Source: CAD feature listing. Evaluate the final solid. Frame: model axes, mm. Give positions to 0.01 mm unless a question says otherwise; leave off trailing zeros. Loops run counter-clockwise (first coordinate to the right, second up) from the corner with the lowest first, then second, coordinate; pieces in that order, holes last. Notation, with made-up numbers: M 44.5,13.5 L 55.5,13.5 A16 ccw 55.5,32.5 Z; hole C 7,71.5 d1. An arc over 180 degrees is marked long. Answer in a Markdown table with one row per item.
```python
from build123d import *

# Parameters (mm, degrees)
EXTRUDE_THIN2_DEPTH = 222.25
FILLET1_R           = 1.27


with BuildPart() as part:
    # Sketch1 → Extrude-Thin2 (new body)
    with BuildSketch(Plane.XY):
        with BuildLine():
            Line((0, 22.225), (-5.55625, 22.225))
            ThreePointArc((-5.55625, 22.225), (-8.727268782, 18.891050689), (-5.23875, 15.890914887))
            Line((-5.23875, 15.890914887), (-5.23875, 12.715914887))
            Line((-5.23875, 12.715914887), (-1.27, 12.715914887))
            Line((-1.27, 12.715914887), (-1.27, 5.55625))
            ThreePointArc((-1.27, 5.55625), (-4.048125, 2.778125), (-1.27, 0))
            Line((-1.27, 0), (0, 0))
            Line((0, 0), (0, 1.27))
            Line((0, 1.27), (-1.27, 1.27))
            ThreePointArc((-1.27, 1.27), (-2.593079188, 3.501936079), (0, 3.591476717))
            Line((0, 3.591476717), (0, 13.985914887))
            Line((0, 13.985914887), (-3.96875, 13.985914887))
            Line((-3.96875, 13.985914887), (-3.96875, 17.996971629))
            ThreePointArc((-3.96875, 17.996971629), (-7.234797593, 18.1491654), (-5.55625, 20.955))
            Line((-5.55625, 20.955), (0, 20.955))
            Line((0, 20.955), (0, 22.225))
        make_face()
    extrude(amount=-EXTRUDE_THIN2_DEPTH)

    # Fillet1
    fillet1_edges = [part.edges().sort_by_distance(p)[0] for p in [
        (-5.23875, 12.715914887, -111.125),
        (-3.96875, 17.996971629, -111.125),
        (0, 13.985914887, -111.125),
        (0, 3.591476717, -111.125),
    ]]
    fillet(fillet1_edges, radius=FILLET1_R)


solid = part.part
```
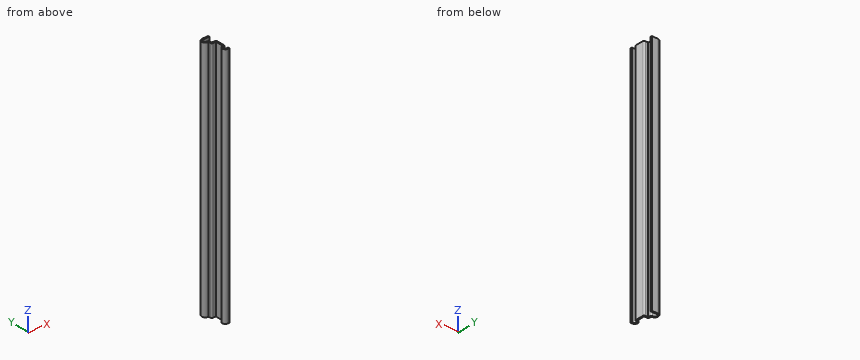
1) Material intervals for L1, parallel to Y at x = -1, z = -159 (3 decimals); L2, parallel to Y at x = -2, z = -200 (3 decimals); L3, parallel to Y at x = -2.5, z = -183 (3 decimals), sorted ascending.
Reply:
| item | result |
|---|---|
| L1 | y = 0 to 1.27, 4.315 to 13.957, 20.955 to 22.225 |
| L2 | y = 0.098 to 1.458, 4.098 to 5.459, 12.716 to 13.986, 20.955 to 22.225 |
| L3 | y = 0.287 to 1.905, 3.651 to 5.269, 12.716 to 13.986, 20.955 to 22.225 |
2) Section B-B, the plane z = -128. Return loops of the section in (x, y) (3 decimals), then the cut area to 3 significant figures.
Reply:
| item | result |
|---|---|
| outline | M -5.556,20.955 L 0,20.955 L 0,22.225 L -5.556,22.225 A3.175 ccw long -5.239,15.891 L -5.239,13.986 A1.27 ccw -3.969,12.716 L -1.27,12.716 L -1.27,5.556 A2.778 ccw -1.27,0 L 0,0 L 0,1.27 L -1.27,1.27 A1.508 cw -1.27,4.286 A1.27 ccw 0,5.556 L 0,12.716 A1.27 ccw -1.27,13.986 L -3.969,13.986 L -3.969,15.891 A1.27 ccw -5.366,17.155 A1.905 cw long Z |
| area | 47.8 mm² |
3) Section A-A, the plane y = 19.05. Return loops of the section in (x, z).
Reply:
| item | result |
|---|---|
| outline | M -8.73,-222.25 L -7.46,-222.25 L -7.46,0 L -8.73,0 Z |
4) Pin query (flat end, axial travel): pin 1 Ø5 at (x, z) = (-7, -182.5) entering from -Y; pin 2 Ø2 at (y, z) = (2.5, -167.5) entering from -X; pin 3 Ø3 at (y, z) = (2.5, -148.5) entering from +X; pin 4 Ø1 at (y, z) = (15, -145.5) entering from -X. Return the tip coordinate at first contact, or that it passes through.
Reply:
| item | result |
|---|---|
| pin 1 | stops at y = 12.83 |
| pin 2 | stops at x = -4.05 |
| pin 3 | stops at x = 0 |
| pin 4 | stops at x = -5.24 |
